Input: dimensioned drawing with shaded views. Units: mm. Origin: part minimum x, y, z. A direction names the side the tool comes from. Give positions to 0.01 mm unless a question says otherwise; leave off trailing zeros. Order: outer loops, then holes, each group sorted by start corner. A loop starts at its lowest first (then second) coordinate and runs counter-clockwise, first axis right, second up.
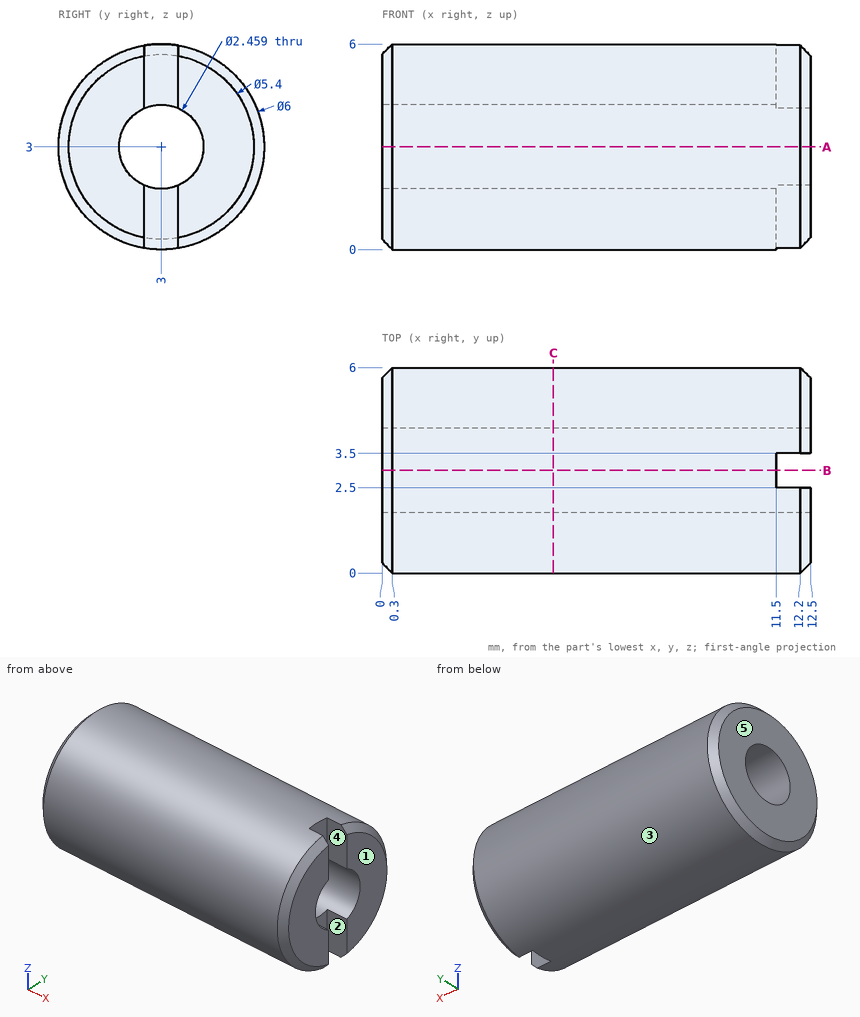
1) Reachability of the marked faces 4 and 5 from +Z, -Z, +X, -X, +Y, -Y: full face, straight path, thin tool, end or side. Return the list, or none.
2) Cut plane C-C (x = 5). Return the cut outline in (y, z), then the cut area to 3 significant figures.
3) Line query: probe 1 along Y at (x, z) = (4, 3); probe 2 along Y at (x, z) = (6.25, 3.5); probe 3 along Z at (x, y) = (5.5, 4). Output: solid intervals per line, ascending.
4) Cut plane B-B (y = 3). Return the cut outline in (x, z), then the cut area to 3 significant figures.
5) Cut plane A-A (z = 3). Return the cut outline in (x, y), then the cut area to 3 significant figures.
6) Pull-direction query (Y, two-part tool) for the marked faces 1, 2 and 3; classes: pulls with the +Y half, pulls with the -Y half, needs draft (parallel to the pull), parting line crosses it, or undercut.
7) First-contact query: P1, Ø0.5, axis at x = 12, z = 5, coming from the +Y side; P2, Ø2, axis at y = 3, z = 3, coming from the +X side; P3, Ø0.5, axis at y = 3, z = 1, coming from the +X side; P4, Ø2, axis at x = 3.5, z = 4.5, coming from the -Y side. Flat tips, straight axial feed; report the tip coordinate or a pass-through.
Geometry says:
1. face 4: +Z, -Z, +X
1. face 5: +Z, -Z, -X, +Y, -Y
2. outline: circle Ø6 at (3, 3); hole circle Ø2.46 at (3, 3)
2. area: 23.5 mm2
3. probe 1: y = 0 to 1.77, 4.23 to 6
3. probe 2: y = 0.04 to 1.88, 4.12 to 5.96
3. probe 3: z = 0.17 to 2.28, 3.72 to 5.83
4. outline: (0, 0.3) - (0.3, 0) - (11.5, 0) - (11.5, 1.77) - (0, 1.77) - close; (0, 4.23) - (11.5, 4.23) - (11.5, 6) - (0.3, 6) - (0, 5.7) - close
4. area: 40.6 mm2
5. outline: (0, 0.3) - (0.3, 0) - (12.2, 0) - (12.5, 0.3) - (12.5, 1.77) - (0, 1.77) - close; (0, 4.23) - (12.5, 4.23) - (12.5, 5.7) - (12.2, 6) - (0.3, 6) - (0, 5.7) - close
5. area: 44.1 mm2
6. face 1: needs draft
6. face 2: undercut
6. face 3: parting line crosses it
7. P1: stops at y = 5.44
7. P2: passes through
7. P3: stops at x = 11.5
7. P4: stops at y = 0.04
